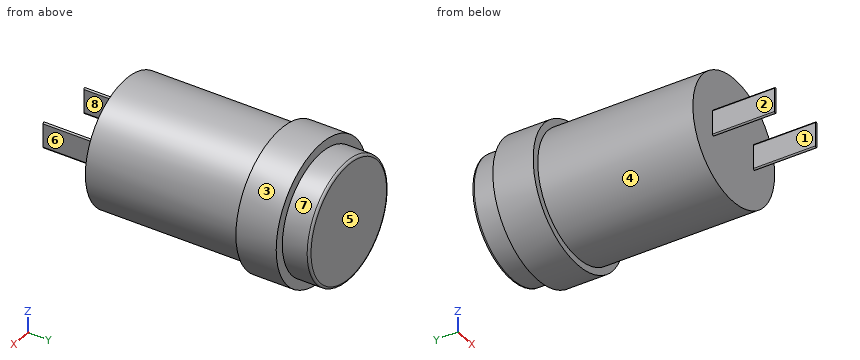
```python
from build123d import *

# Parameters (mm, degrees)
SKETCH1_R           = 8.9
BOSS_EXTRUDE1_DEPTH = 5.2
SKETCH2_R           = 8
BOSS_EXTRUDE2_DEPTH = 20
BOSS_EXTRUDE3_DEPTH = 8
SKETCH4_R           = 7.7
BOSS_EXTRUDE4_DEPTH = 3.5
FILLET1_R           = 0.3
SCALE1_SCALE        = 1.375


with BuildPart() as part:
    # Sketch1 → Boss-Extrude1 (new body)
    with BuildSketch(Plane(origin=(0, 0, 0), x_dir=(1, 0, 0), z_dir=(0, 1, 0))):
        Circle(SKETCH1_R)
    extrude(amount=BOSS_EXTRUDE1_DEPTH)

    # Sketch2 → Boss-Extrude2 (add)
    with BuildSketch(Plane.XZ):
        Circle(SKETCH2_R)
    extrude(amount=BOSS_EXTRUDE2_DEPTH)

    # Sketch3 → Boss-Extrude3 (add)
    with BuildSketch(Plane.XZ.offset(20)):
        with BuildLine():
            Line((4.15, 1.5), (4.15, -1.5))
            ThreePointArc((4.15, -1.5), (4, -1.65), (3.85, -1.5))
            Line((3.85, -1.5), (3.85, 1.5))
            ThreePointArc((3.85, 1.5), (4, 1.65), (4.15, 1.5))
        make_face()
        with BuildLine():
            Line((-3.85, 1.5), (-3.85, -1.5))
            ThreePointArc((-3.85, -1.5), (-4, -1.65), (-4.15, -1.5))
            Line((-4.15, -1.5), (-4.15, 1.5))
            ThreePointArc((-4.15, 1.5), (-4, 1.65), (-3.85, 1.5))
        make_face()
    extrude(amount=BOSS_EXTRUDE3_DEPTH)

    # Sketch4 → Boss-Extrude4 (add)
    with BuildSketch(Plane(origin=(0, 5.2, 0), x_dir=(1, 0, 0), z_dir=(0, 1, 0))):
        Circle(SKETCH4_R)
    extrude(amount=BOSS_EXTRUDE4_DEPTH)

    # Fillet1
    fillet1_edges = [part.edges().sort_by_distance(p)[0] for p in [
        (-7.7, 8.7, 0),
    ]]
    fillet(fillet1_edges, radius=FILLET1_R)


with BuildPart() as part_1:
    # Scale1: scaled about (0, -5.466249854, 0)
    add(part.part.scale(SCALE1_SCALE).moved(Location((0, 2.049843695, 0))))


solid = part_1.part
```
Model file for the job. Use its own axes, mm. Face numbers are marked on the shaded views. A direction names the side the tool comes from. Coordinates: 2 decimals unless noted, no trailing zeros. Loops run counter-clockwise (first coordinate to the right, second up) from the corner with the lowest first, then second, coordinate; pieces in that order, holes last. Notation, with made-up numbers: (56.25, 29.25) - (62.25, 29.25) arc R17 cw to (62.25, 60.25) - close; hole circle Ø6 at (-16, -1.5). An arc over 180 degrees is marked (long way). Write item = value, one per line. Start each with the question number.
Item 1: Wall check: probe 1 along X at (y, z) = (-30, -0.25); probe 2 along Y at (x, z) = (-3.75, 1.5); probe 3 along Y at (x, z) = (0.25, 11.25). Give the ranges that are in metal, low to high. Write a range as [from, to].
Item 2: Drop flat-ended pins along their axis: pin 1 Ø1.2 at (y, z) = (-32, 0.5) entering from +X; pin 2 Ø1 at (y, z) = (4, -5) entering from +X; pin 3 Ø1 at (y, z) = (-6.5, 9.5) entering from -X. Give the stop position or say it passes through.
Item 3: Pull direction X, two halves, no side cores. Call the marked faces 5, 6, 7 and 8: +X half, -X half, draft (parallel to the pull), parting line (faces both ways), or undercut.
Item 4: Saw through at B-B, the plane y = -16.5. List the corners of the cut face in (x, z).
Item 5: 3-axis set-ups, long thin cutter, end or side, ignore diameter. For the marked faces 1, 2, 3 and 4: which of +Z, -Z, +X, -X, +Y, -Y reach the whole face in a straight line?
Item 6: Saw through at A-A, the plane x = 0. List the corners of the cut face in (y, z) (1 decimal), then the cut area to 3 significant figures.
Answers:
q1.probe_1 = [-5.71, -5.29], [5.29, 5.71]
q1.probe_2 = [-25.45, 14.01]
q1.probe_3 = [2.05, 9.2]
q2.pin_1 = 5.71
q2.pin_2 = 11.38
q2.pin_3 = -6.32
q3.face_5 = draft
q3.face_6 = +X half
q3.face_7 = parting line
q3.face_8 = undercut
q4.outline = circle Ø22 at (0, 0)
q5.face_1 = +Z, -Z, -Y
q5.face_2 = +Z, -Z, -X, -Y
q5.face_3 = +Y, -Y
q5.face_4 = -Y
q6.outline = (-25.5, -11) - (2, -11) - (2, -12.2) - (9.2, -12.2) - (9.2, -10.6) - (13.6, -10.6) arc R0.4 ccw to (14, -10.2) - (14, 10.2) arc R0.4 ccw to (13.6, 10.6) - (9.2, 10.6) - (9.2, 12.2) - (2, 12.2) - (2, 11) - (-25.5, 11) - close
q6.area = 882 mm2
